```python
from build123d import *

# Parameters (mm, degrees)
F0_W     = 23.546827
F0_H     = 25.524346
F1_DEPTH = 12
F3_D     = 5
F6_D     = 5.08


with BuildPart() as f1:
    # F0 (on Front) → F1 (new body)
    with BuildSketch(Plane.XZ):
        with Locations((-16.37222, 12.762173)):
            Rectangle(F0_W, F0_H)
    extrude(amount=F1_DEPTH)

    # F3 (through all)
    with Locations(Plane.XY.offset(25.524346)):
        with Locations((-24.82892, -6.173369)):
            Hole(F3_D / 2)

    # F6 (through all)
    with Locations(Plane.XZ.offset(12)):
        with Locations((-11.741878, 11.862813)):
            Hole(F6_D / 2)


solid = f1.part
```
Can you work these out from the model? Positions are in its coordinate system, mm. Coordinates: 2 decimals unless noted, no trailing zeros. Order: outer loops, then holes, each group sorted by start corner. A loop starts at its lowest first (then second) coordinate and runs counter-clockwise, first axis right, second up. Notation, with made-up numbers: (11, 32) -> (43, 32) arc R12 cw to (43, 49) -> close; hole circle Ø5 at (15, 3). An arc over 180 degrees is marked (long way). Write each question's results on one line, items separated by ' | '.
Item 1: If we mould it in two halves opening along Y, with no side actions, what happens to faces 1 (the face through (-22.33, -6.06, 12.58)), 2 (the face through (-28.146, -6, 13)), 3 (the face through (-17, -12, 13)), 4 (the face through (-17, 0, 13))? For each: +Y half, -Y half, draft (parallel to the pull), parting line (faces both ways), or undercut.
Results are:
face 1: undercut | face 2: draft | face 3: -Y half | face 4: +Y half
Item 2: If I drill on line 1 along Z through (x, y) = (-13.5, -11.25); line 2 along Z through (x, y) = (-10.75, -7); line 3 along X through (y, z) = (-5, 23.5), over which ranges is the centre line in solid material (lowest first)?
Results are:
line 1: 0 to 10.03, 13.7 to 25.52 | line 2: 0 to 9.52, 14.2 to 25.52 | line 3: -28.15 to -27.04, -22.62 to -4.6
Item 3: I want a section at B-B, the plane z = 12.5. Write out the boundary of the cut face in (x, y), then the cut area to 3 significant figures.
Results are:
outline: (-28.15, -12) -> (-14.2, -12) -> (-14.2, 0) -> (-28.15, 0) -> close; (-9.28, -12) -> (-4.6, -12) -> (-4.6, 0) -> (-9.28, 0) -> close; hole circle Ø5 at (-24.83, -6.17) | area: 204 mm²
Item 4: I want a section at C-C, the plane x = -11.5. Write out the boundary of the cut face in (y, z).
Results are:
outline: (-12, 0) -> (0, 0) -> (0, 9.33) -> (-12, 9.33) -> close; (-12, 14.39) -> (0, 14.39) -> (0, 25.52) -> (-12, 25.52) -> close
Item 5: I want a section at D-D, the plane y = -2. Write out the boundary of the cut face in (x, z).
Results are:
outline: (-28.15, 0) -> (-4.6, 0) -> (-4.6, 25.52) -> (-28.15, 25.52) -> close; hole circle Ø5.08 at (-11.74, 11.86)
Item 6: I want a section at A-A, the plane y = -5.5. Write out the boundary of the cut face in (x, z).
Results are:
outline: (-28.15, 0) -> (-27.24, 0) -> (-27.24, 25.52) -> (-28.15, 25.52) -> close; (-22.42, 0) -> (-4.6, 0) -> (-4.6, 25.52) -> (-22.42, 25.52) -> close; hole circle Ø5.08 at (-11.74, 11.86)
